Input: dimensioned drawing with shaded views. Units: mm. Origin: part minimum x, y, z. A direction names the side the tool comes from. Coordinates: 2 decimals unless noted, no trailing zeros. Loops run counter-clockwise (first coordinate to the right, second up) from the corner with the lowest first, then second, coordinate; pieces in that order, holes last. Notation, with made-up numbers: (89, 4.5) -> (98, 4.5) arc R32 ccw to (98, 41.5) -> close; hole circle Ø1 at (-1.75, 79). An arc over 180 degrees is marked (long way). Answer as CSV lines item,"result".
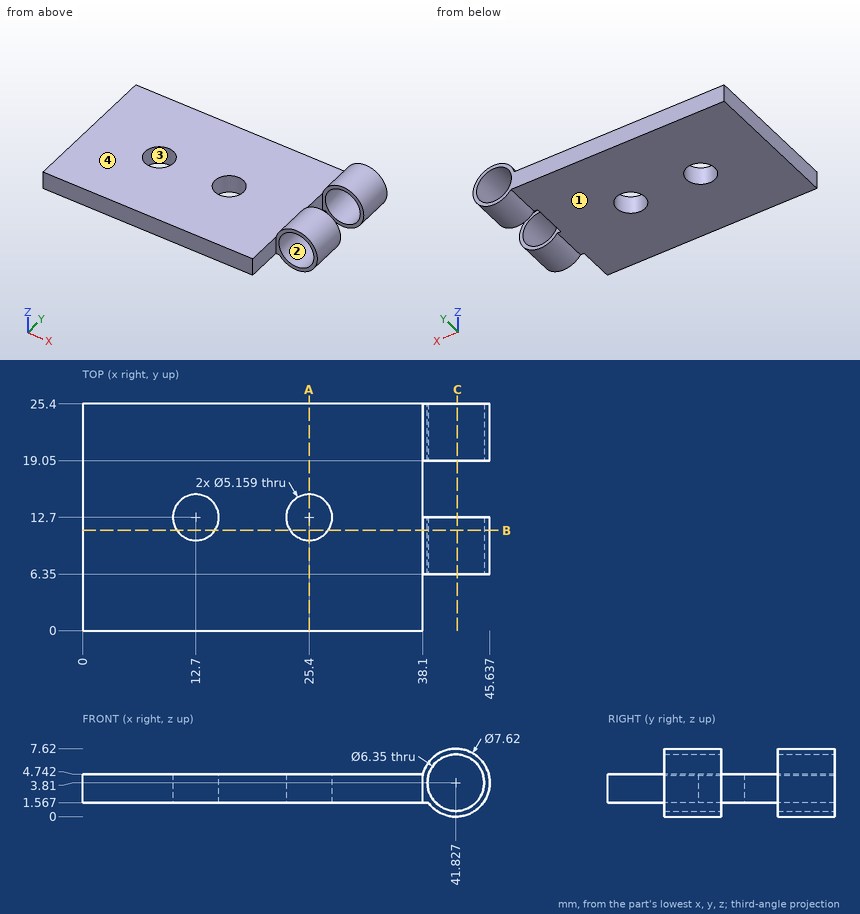
(1) Pin query (flat end, axial travel): pin 1 Ø12 at (x, y) = (34, 21) entering from +Z; pin 2 Ø7.5 at (x, y) = (28.5, 16.5) entering from -Z. Return the tip coordinate at first contact, or that it passes through.
Computed values:
pin 1,"z = 7.15"
pin 2,"z = 1.57"
(2) Draft query along X for the marked faces 1 and 2. Return one class per face: released by +X, released by -X, zero draft, split by the parting line, or undercut.
Computed values:
face 1,"zero draft"
face 2,"undercut"
(3) Access query for the marked faces 3 and 4. Directions: +Z, -Z, +X, -X, +Y, -Y. A direction counts if a zero-diameter tool reaches every point of the face in a straight line with its end or side. Return the directions, or none.
Computed values:
face 3,"+Z, -Z"
face 4,"+Z, -X, +Y, -Y"
(4) Cut plane A-A (x = 25.4). Return the cut outline in (y, z).
Computed values:
outline,"(0, 1.57) -> (10.12, 1.57) -> (10.12, 4.74) -> (0, 4.74) -> close; (15.28, 1.57) -> (25.4, 1.57) -> (25.4, 4.74) -> (15.28, 4.74) -> close"
(5) Material intervals for L1, parallel to Y at x = 25.4, z = 3.25; L2, parallel to Z at x = 25.5, y = 17.25; L3, parallel to X at y = 13.5, z = 1.75, sorted ascending. Write a range as [from, to].
Computed values:
L1,"[0, 10.12], [15.28, 25.4]"
L2,"[1.57, 4.74]"
L3,"[0, 10.25], [15.15, 22.95], [27.85, 38.1]"
(6) Cut plane B-B (y = 11.25). State how many separate pieces and enclosed holes the cut face has, then the cut area to 3 significant figures.
Computed values:
separate pieces,"3"
enclosed holes,"1"
area,"108 mm^2"
(7) Cut plane C-C (x = 42). Return the cut outline in (y, z).
Computed values:
outline,"(6.35, 0) -> (12.7, 0) -> (12.7, 0.64) -> (6.35, 0.64) -> close; (6.35, 6.98) -> (12.7, 6.98) -> (12.7, 7.62) -> (6.35, 7.62) -> close; (19.05, 0) -> (25.4, 0) -> (25.4, 0.64) -> (19.05, 0.64) -> close; (19.05, 6.98) -> (25.4, 6.98) -> (25.4, 7.62) -> (19.05, 7.62) -> close"
